Job drawing, mm, ordinate dimensions from the low corner. One solid piece. A direction names the side the tool comes from. Coordinates: 2 decimals unless noted, no trailing zeros. Loops run counter-clockwise (first coordinate to the right, second up) from the corner with the lowest first, then second, coordinate; pieces in that order, holes last. Notation, with made-up numbers: (-33.75, -13) -> (12.25, -13) arc R26 ccw to (12.25, 4) -> close; hole circle Ø3 at (22.5, 55). An arc over 180 degrees is marked (long way). Answer as CSV lines item,"result". Start each with the question number.
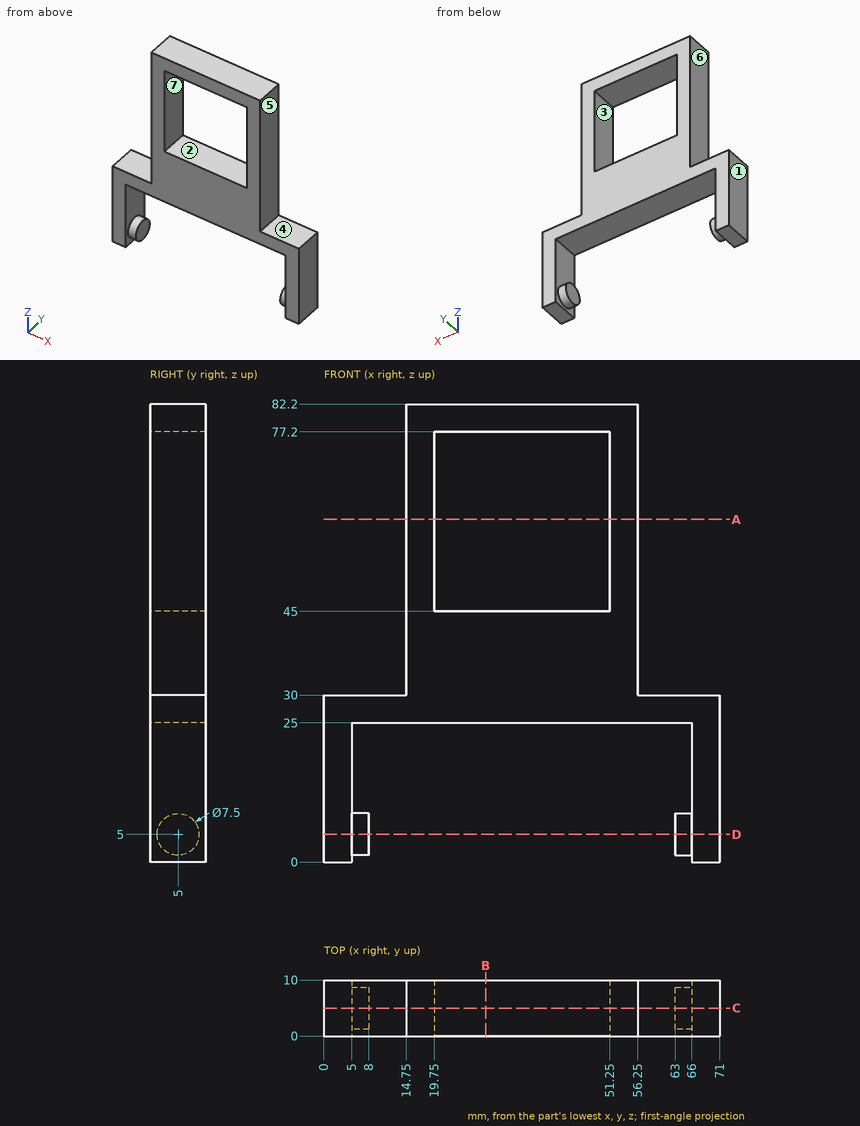
Item 1: Wall check: probe 1 along Z at (x, y) = (41.5, 3.75); probe 2 along X at (y, z) = (4.25, 52.5); probe 3 along X at (y, z) = (5, 15.5). Give the ranges that are in metal, low to high.
Item 2: Flat gauge pins, fed straight in: pin 1 Ø1.5 at (x, y) = (8, 3.5) entering from +Z; pin 2 Ø1 at (y, z) = (5, 62) entering from +X; pin 3 Ø6 at (x, y) = (32.5, 5) entering from -Z. Where does each tip first touch, or does it go through?
Item 3: Saw through at B-B (x = 29). Write the cut outline in (y, z).
Item 4: Two-plate mould, pull along Z, no slides. Class the marked faces 1, 2, 3 and 4: pulls with the +Z half, pulls with the -Z half, needs draft (parallel to the pull), parting line crosses it, or undercut.
Item 5: Saw through at D-D (z = 5). Write the cut outline in (x, y).
Item 6: Saw through at C-C (y = 5). Write the cut outline in (x, z).
Item 7: Saw through at A-A (z = 61.5). Write the cut outline in (x, y).
Item 8: Which spindle directions (+Z, -Z, +X, -X, +Y, -Y) get a long thin tool onto all of the face, cutting with end or side? Do the marked faces 5, 6 and 7. Say none if no direction does.
Geometry check:
1,probe 1,"25 to 45, 77.2 to 82.2"
1,probe 2,"14.75 to 19.75, 51.25 to 56.25"
1,probe 3,"0 to 5, 66 to 71"
2,pin 1,"z = 30"
2,pin 2,"x = 56.25"
2,pin 3,"z = 25"
3,outline,"(0, 25) -> (10, 25) -> (10, 45) -> (0, 45) -> close; (0, 77.2) -> (10, 77.2) -> (10, 82.2) -> (0, 82.2) -> close"
4,face 1,"needs draft"
4,face 2,"undercut"
4,face 3,"undercut"
4,face 4,"pulls with the +Z half"
5,outline,"(0, 0) -> (5, 0) -> (5, 1.25) -> (8, 1.25) -> (8, 8.75) -> (5, 8.75) -> (5, 10) -> (0, 10) -> close; (63, 1.25) -> (66, 1.25) -> (66, 0) -> (71, 0) -> (71, 10) -> (66, 10) -> (66, 8.75) -> (63, 8.75) -> close"
6,outline,"(0, 0) -> (5, 0) -> (5, 1.25) -> (8, 1.25) -> (8, 8.75) -> (5, 8.75) -> (5, 25) -> (66, 25) -> (66, 8.75) -> (63, 8.75) -> (63, 1.25) -> (66, 1.25) -> (66, 0) -> (71, 0) -> (71, 30) -> (56.25, 30) -> (56.25, 82.2) -> (14.75, 82.2) -> (14.75, 30) -> (0, 30) -> close; hole (19.75, 45) -> (51.25, 45) -> (51.25, 77.2) -> (19.75, 77.2) -> close"
7,outline,"(14.75, 0) -> (19.75, 0) -> (19.75, 10) -> (14.75, 10) -> close; (51.25, 0) -> (56.25, 0) -> (56.25, 10) -> (51.25, 10) -> close"
8,face 5,"+Z, +X, +Y, -Y"
8,face 6,"+Z, -X, +Y, -Y"
8,face 7,"+Y, -Y"
